```python
from build123d import *

# Parameters (mm, degrees)
SKETCH1_W               = 200
SKETCH1_H               = 120
BOSS_EXTRUDE1_DEPTH     = 3
SKETCH2_W               = 120
SKETCH2_H               = 50
BOSS_EXTRUDE2_DEPTH     = 8
SKETCH3_W               = 116
SKETCH3_H               = 1
SKETCH3_H_2             = 6
CUT_EXTRUDE2_DEPTH      = 48
SKETCH4_W               = 25
SKETCH4_H               = 10.416666666
CUT_EXTRUDE3_DEPTH      = 4
CUT_EXTRUDE4_DEPTH      = 4
FILLET1_R               = 20
SKETCH6_W               = 15
SKETCH6_H               = 7.5
BOSS_EXTRUDE3_DEPTH     = 10
SKETCH7_W               = 2.5
SKETCH7_H               = 7.5
CUT_EXTRUDE5_DEPTH      = 17
FILLET4_R               = 2
FILLET5_R               = 5
CUT_EXTRUDE6_DEPTH      = 10
FILLET4_OF_MIRROR3_R    = 2
FILLET5_OF_MIRROR3_R    = 5
SKETCH10_R              = 2.5
CUT_EXTRUDE7_DEPTH      = 15
MIRROR5_COPY_1_SKETCH_R = 2.5
MIRROR5_COPY_1_DEPTH    = 15


with BuildPart() as part:
    # Sketch1 → Boss-Extrude1 (new body)
    with BuildSketch(Plane(origin=(0, 0, 0), x_dir=(1, 0, 0), z_dir=(0, 1, 0))):
        Rectangle(SKETCH1_W, SKETCH1_H)
    extrude(amount=BOSS_EXTRUDE1_DEPTH)

    # Sketch2 → Boss-Extrude2 (add)
    with BuildSketch(Plane.XZ):
        Rectangle(SKETCH2_W, SKETCH2_H)
    extrude(amount=BOSS_EXTRUDE2_DEPTH)

    # Sketch3 → Cut-Extrude2 (cut)
    with BuildSketch(Plane.XY.offset(25)):
        with Locations((0, -0.5)):
            Rectangle(SKETCH3_W, SKETCH3_H)
        with Locations((0, -4)):
            Rectangle(SKETCH3_W, SKETCH3_H_2)
    extrude(amount=-CUT_EXTRUDE2_DEPTH, mode=Mode.SUBTRACT)

    # Sketch4 → Cut-Extrude3 (cut)
    with BuildSketch(Plane(origin=(0, 3, 0), x_dir=(1, 0, 0), z_dir=(0, 1, 0))):
        Polygon((12.5, -8), (42.5, -22), (-42.5, -22), (-12.5, -8), align=None)
        Polygon((56, 20), (56, -20), (16, -4), (16, 4), align=None)
        Polygon((-12.5, 8), (12.5, 8), (42.5, 22), (-42.5, 22), align=None)
        Rectangle(SKETCH4_W, SKETCH4_H)
        Polygon((-16, -4), (-16, 0), (-56, 0), (-56, -20), align=None)
        Polygon((-16, 0), (-16, 4), (-56, 20), (-56, 0), align=None)
    extrude(amount=-CUT_EXTRUDE3_DEPTH, mode=Mode.SUBTRACT)

    # Sketch5 → Cut-Extrude4 (cut)
    with BuildSketch(Plane.XZ.offset(8)):
        with BuildLine():
            Line((9, 20), (9, -20))
            ThreePointArc((9, -20), (9.585786438, -21.414213562), (11, -22))
            Line((11, -22), (13, -22))
            ThreePointArc((13, -22), (14.414213562, -21.414213562), (15, -20))
            Line((15, -20), (15, 20))
            ThreePointArc((15, 20), (14.414213562, 21.414213562), (13, 22))
            Line((13, 22), (11, 22))
            ThreePointArc((11, 22), (9.585786438, 21.414213562), (9, 20))
        make_face()
        with BuildLine():
            Line((-1, 22), (1, 22))
            ThreePointArc((1, 22), (2.414213562, 21.414213562), (3, 20))
            Line((3, 20), (3, -20))
            ThreePointArc((3, -20), (2.414213562, -21.414213562), (1, -22))
            Line((1, -22), (-1, -22))
            ThreePointArc((-1, -22), (-2.414213562, -21.414213562), (-3, -20))
            Line((-3, -20), (-3, 20))
            ThreePointArc((-3, 20), (-2.414213562, 21.414213562), (-1, 22))
        make_face()
        with BuildLine():
            Line((21, 20), (21, -20))
            ThreePointArc((21, -20), (21.585786438, -21.414213562), (23, -22))
            Line((23, -22), (25, -22))
            ThreePointArc((25, -22), (26.414213562, -21.414213562), (27, -20))
            Line((27, -20), (27, 20))
            ThreePointArc((27, 20), (26.414213562, 21.414213562), (25, 22))
            Line((25, 22), (23, 22))
            ThreePointArc((23, 22), (21.585786438, 21.414213562), (21, 20))
        make_face()
        with BuildLine():
            Line((33, 20), (33, -20))
            ThreePointArc((33, -20), (33.585786438, -21.414213562), (35, -22))
            Line((35, -22), (37, -22))
            ThreePointArc((37, -22), (38.414213562, -21.414213562), (39, -20))
            Line((39, -20), (39, 20))
            ThreePointArc((39, 20), (38.414213562, 21.414213562), (37, 22))
            Line((37, 22), (35, 22))
            ThreePointArc((35, 22), (33.585786438, 21.414213562), (33, 20))
        make_face()
        with BuildLine():
            Line((45, 20), (45, -20))
            ThreePointArc((45, -20), (45.585786438, -21.414213562), (47, -22))
            Line((47, -22), (49, -22))
            ThreePointArc((49, -22), (50.414213562, -21.414213562), (51, -20))
            Line((51, -20), (51, 20))
            ThreePointArc((51, 20), (50.414213562, 21.414213562), (49, 22))
            Line((49, 22), (47, 22))
            ThreePointArc((47, 22), (45.585786438, 21.414213562), (45, 20))
        make_face()
        with BuildLine():
            Line((-15, 20), (-15, -20))
            ThreePointArc((-15, -20), (-14.414213562, -21.414213562), (-13, -22))
            Line((-13, -22), (-11, -22))
            ThreePointArc((-11, -22), (-9.585786438, -21.414213562), (-9, -20))
            Line((-9, -20), (-9, 20))
            ThreePointArc((-9, 20), (-9.585786438, 21.414213562), (-11, 22))
            Line((-11, 22), (-13, 22))
            ThreePointArc((-13, 22), (-14.414213562, 21.414213562), (-15, 20))
        make_face()
        with BuildLine():
            Line((-27, 20), (-27, -20))
            ThreePointArc((-27, -20), (-26.414213562, -21.414213562), (-25, -22))
            Line((-25, -22), (-23, -22))
            ThreePointArc((-23, -22), (-21.585786438, -21.414213562), (-21, -20))
            Line((-21, -20), (-21, 20))
            ThreePointArc((-21, 20), (-21.585786438, 21.414213562), (-23, 22))
            Line((-23, 22), (-25, 22))
            ThreePointArc((-25, 22), (-26.414213562, 21.414213562), (-27, 20))
        make_face()
        with BuildLine():
            Line((-39, 20), (-39, -20))
            ThreePointArc((-39, -20), (-38.414213562, -21.414213562), (-37, -22))
            Line((-37, -22), (-35, -22))
            ThreePointArc((-35, -22), (-33.585786438, -21.414213562), (-33, -20))
            Line((-33, -20), (-33, 20))
            ThreePointArc((-33, 20), (-33.585786438, 21.414213562), (-35, 22))
            Line((-35, 22), (-37, 22))
            ThreePointArc((-37, 22), (-38.414213562, 21.414213562), (-39, 20))
        make_face()
        with BuildLine():
            Line((-51, 20), (-51, -20))
            ThreePointArc((-51, -20), (-50.414213562, -21.414213562), (-49, -22))
            Line((-49, -22), (-47, -22))
            ThreePointArc((-47, -22), (-45.585786438, -21.414213562), (-45, -20))
            Line((-45, -20), (-45, 20))
            ThreePointArc((-45, 20), (-45.585786438, 21.414213562), (-47, 22))
            Line((-47, 22), (-49, 22))
            ThreePointArc((-49, 22), (-50.414213562, 21.414213562), (-51, 20))
        make_face()
    extrude(amount=-CUT_EXTRUDE4_DEPTH, mode=Mode.SUBTRACT)

    # Fillet1
    fillet1_edges = [part.edges().sort_by_distance(p)[0] for p in [
        (100, 1.5, 60),
        (-100, 1.5, 60),
        (-100, 1.5, -60),
        (100, 1.5, -60),
    ]]
    fillet(fillet1_edges, radius=FILLET1_R)

    # Sketch6 → Boss-Extrude3 (add)
    with BuildSketch(Plane(origin=(0, 3, 0), x_dir=(1, 0, 0), z_dir=(0, 1, 0))):
        with Locations((-47.5, 56.25)):
            Rectangle(SKETCH6_W, SKETCH6_H)
    boss_extrude3 = extrude(amount=BOSS_EXTRUDE3_DEPTH)

    # Sketch7 → Cut-Extrude5 (cut)
    with BuildSketch(Plane.ZY.offset(55)):
        with Locations((-53.75, 6.75)):
            Rectangle(SKETCH7_W, SKETCH7_H)
    cut_extrude5 = extrude(amount=-CUT_EXTRUDE5_DEPTH, mode=Mode.SUBTRACT)

    # Fillet4
    fillet4_edges = [part.edges().sort_by_distance(p)[0] for p in [
        (-47.5, 3, -55),
    ]]
    fillet(fillet4_edges, radius=FILLET4_R)

    # Fillet5
    fillet5_edges = [part.edges().sort_by_distance(p)[0] for p in [
        (-47.5, 13, -60),
    ]]
    fillet(fillet5_edges, radius=FILLET5_R)

    # Sketch8 → Cut-Extrude6 (cut)
    with BuildSketch(Plane(origin=(0, 3, 0), x_dir=(1, 0, 0), z_dir=(0, 1, 0))):
        with BuildLine():
            Line((-58, 34.5), (58, 34.5))
            ThreePointArc((58, 34.5), (59.414213562, 33.914213562), (60, 32.5))
            Line((60, 32.5), (60, 31.5))
            ThreePointArc((60, 31.5), (59.414213562, 30.085786438), (58, 29.5))
            Line((58, 29.5), (-58, 29.5))
            ThreePointArc((-58, 29.5), (-59.414213562, 30.085786438), (-60, 31.5))
            Line((-60, 31.5), (-60, 32.5))
            ThreePointArc((-60, 32.5), (-59.414213562, 33.914213562), (-58, 34.5))
        make_face()
    cut_extrude6 = extrude(amount=-CUT_EXTRUDE6_DEPTH, mode=Mode.SUBTRACT)

    # Mirror1: Cut-Extrude6 across plane
    add(cut_extrude6.mirror(Plane.XY), mode=Mode.SUBTRACT)

    # Mirror3: Boss-Extrude3, Cut-Extrude5 across plane
    add(boss_extrude3.mirror(Plane(origin=(0, 0, 0), x_dir=(0, 0, 1), z_dir=(1, 0, 0))))
    add(cut_extrude5.mirror(Plane(origin=(0, 0, 0), x_dir=(0, 0, 1), z_dir=(1, 0, 0))), mode=Mode.SUBTRACT)

    # Fillet4 of Mirror3
    fillet4_of_mirror3_edges = [part.edges().sort_by_distance(p)[0] for p in [
        (47.5, 3, -55),
    ]]
    fillet(fillet4_of_mirror3_edges, radius=FILLET4_OF_MIRROR3_R)

    # Fillet5 of Mirror3
    fillet5_of_mirror3_edges = [part.edges().sort_by_distance(p)[0] for p in [
        (47.5, 13, -60),
    ]]
    fillet(fillet5_of_mirror3_edges, radius=FILLET5_OF_MIRROR3_R)

    # Sketch10 → Cut-Extrude7 (cut)
    with BuildSketch(Plane(origin=(0, 3, 0), x_dir=(1, 0, 0), z_dir=(0, 1, 0))):
        with Locations(Location((85, -45, 0), (0, 0, 270))):
            Circle(SKETCH10_R)
    cut_extrude7 = extrude(amount=-CUT_EXTRUDE7_DEPTH, mode=Mode.SUBTRACT)

    # Mirror4: Cut-Extrude7 across plane
    add(cut_extrude7.mirror(Plane(origin=(0, 0, 0), x_dir=(0, 0, 1), z_dir=(1, 0, 0))), mode=Mode.SUBTRACT)

    # Mirror5: Cut-Extrude7 across plane
    add(cut_extrude7.mirror(Plane.XY), mode=Mode.SUBTRACT)

    # Mirror5 copy 1 sketch → Mirror5 copy 1 (cut)
    with BuildSketch(Plane(origin=(0, 3, 0), x_dir=(-1, 0, 0), z_dir=(0, 1, 0))):
        with Locations(Location((85, -45, 0), (0, 0, 270))):
            Circle(MIRROR5_COPY_1_SKETCH_R)
    extrude(amount=-MIRROR5_COPY_1_DEPTH, mode=Mode.SUBTRACT)


solid = part.part
```
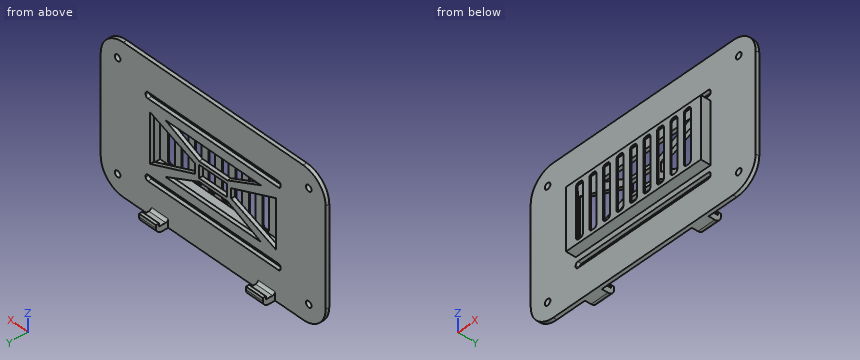
Could you check a few things on this model? Use its own coordinates, in mm. Round coordinates to 2 decimals unless told otherwise and drop trailing zeros. Write each loop counter-clockwise with the first axis right and the second up, starting at its lowest first coordinate (ties: lowest second). Pieces come first, ordered by that corner, then holes. Notation, with made-up numbers: M 9,64.5 L 43,64.5 A24 ccw 43,99.5 Z; hole C 19.25,36 d6. An arc over 180 degrees is marked long. Answer in a Markdown table with one row per item. Add a question column.
Q1. Imagine slicing it at C-C (z = 45). Please give me the cut outline in (x, y), then the cut area to 3 significant figures.
Q2. Imagine slicing it at D-D (x = 62.5). Please give me the cut outline in (y, z), then the cut area to 3 significant figures.
Q3. Imagine slicing it at A-A (x = -6.5). Give the number of separate pieces and of enclosed holes in the cut face, then the cut area to 3 significant figures.
Q4. If I drill on line 1 (Y direction, x = -20.5, z = 24); line 2 (X direction, y = 1.3, z = -45); line 3 (Y direction, x = 65.5, z = -44), over which ranges is the centre line in solid material (lowest first)? Write a range as from..to.
Q5. Imagine slicing it at B-B (x = -85). Please give me the cut outline in (y, z).
Q6. Will these pins go through, and if not, where does the flat tip stop? pin 1 Ø1.1 at (y, z) = (-7.5, -1) entering from -X; pin 2 Ø4 at (y, z) = (-3.5, 48) entering from +X; pin 3 Ø1 at (x, z) = (-4, -4) entering from +Y; pin 4 Ø1.1 at (x, y) = (36, -7.5) entering from +Z.
Values:
| question | item | result |
|---|---|---|
| 1 | outline | M -99.36,0 L -87.5,0 L -87.5,3 L -99.36,3 Z; M -82.5,0 L 82.5,0 L 82.5,3 L -82.5,3 Z; M 87.5,0 L 99.36,0 L 99.36,3 L 87.5,3 Z |
| 1 | area | 566 mm^2 |
| 2 | outline | M 0,-60 L 3,-60 L 3,60 L 0,60 Z |
| 2 | area | 360 mm^2 |
| 3 | separate pieces | 6 |
| 3 | enclosed holes | 0 |
| 3 | area | 279 mm^2 |
| 4 | line 1 | -8..-7, 0..3 |
| 4 | line 2 | -99.36..-87.5, -82.5..82.5, 87.5..99.36 |
| 4 | line 3 | 0..3 |
| 5 | outline | M 0,-59.36 L 3,-59.36 L 3,-47.5 L 0,-47.5 Z; M 0,-42.5 L 3,-42.5 L 3,42.5 L 0,42.5 Z; M 0,47.5 L 3,47.5 L 3,59.36 L 0,59.36 Z |
| 6 | pin 1 | x = -60 |
| 6 | pin 2 | through |
| 6 | pin 3 | y = -7 |
| 6 | pin 4 | z = 25 |
